Input: dimensioned drawing with shaded views. Units: mm. Origin: part minimum x, y, z. Round coordinates to 2 decimals unless told otherwise and drop trailing zeros. Order: outer loops, then holes, each group sorted by start corner. A loop starts at its lowest first (then second) coordinate and runs counter-clockwise, first axis right, second up.
Item 1: Line query: L1, parallel to Y at x = 81, z = 9.75; L2, parallel to X at y = 5.25, z = 7; L3, parallel to Z at x = 9.5, y = 7. Output: solid intervals per line, ascending.
Item 2: Cut plane C-C on x = 91. Output: boundary loops of the cut face in (y, z).
Item 3: Cut plane A-A on x = 5. Output: boundary loops of the cut face in (y, z).
Item 4: Cut plane B-B on z = 6.5. Output: boundary loops of the cut face in (x, y).
Item 5: First-contact query: pin 1 (2.5 mm diameter, centred on x = 91, y = 5, fed in from -Z); pin 2 (3 mm diameter, centred on x = 26.5, y = 7.5, fed in from +Z). Flat tips, straight axial feed; report the tip coordinate or a pass-through.
Item 6: Mould query, pull axis X, two halves, no side actions, for the marked faces 1, 2 and 3. Classes: released by +X, released by -X, zero draft, split by the parting line, or undercut.
Item 7: Cut plane D-D on y = 2.5. Output: boundary loops of the cut face in (x, z).
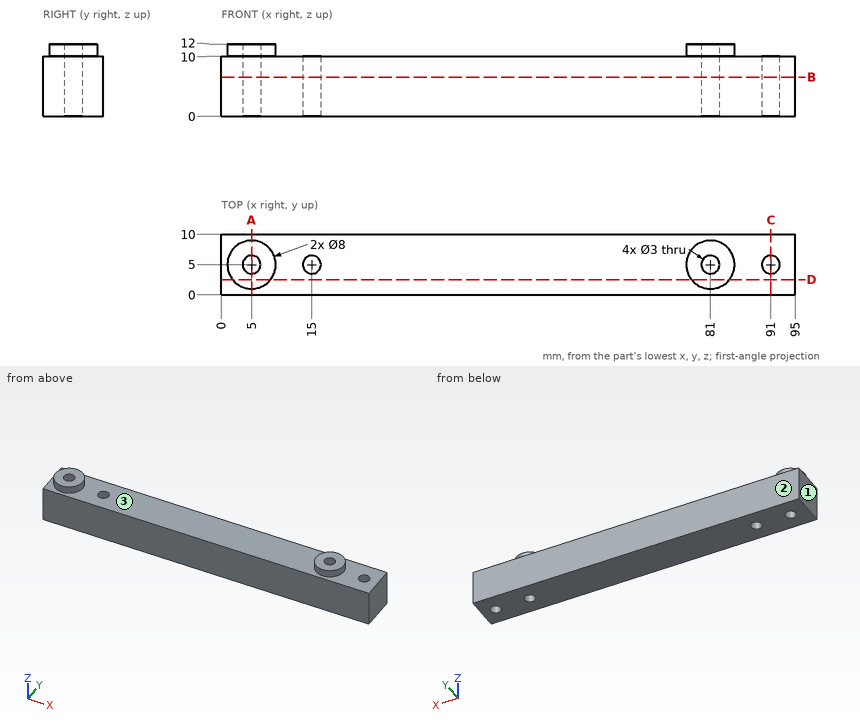
From the geometry:
1. L1: y = 0 to 3.5, 6.5 to 10
1. L2: x = 0 to 3.52, 6.48 to 13.52, 16.48 to 79.52, 82.48 to 89.52, 92.48 to 95
1. L3: z = 0 to 10
2. outline: (0, 0) - (3.5, 0) - (3.5, 10) - (0, 10) - close; (6.5, 0) - (10, 0) - (10, 10) - (6.5, 10) - close
3. outline: (0, 0) - (3.5, 0) - (3.5, 12) - (1, 12) - (1, 10) - (0, 10) - close; (6.5, 0) - (10, 0) - (10, 10) - (9, 10) - (9, 12) - (6.5, 12) - close
4. outline: (0, 0) - (95, 0) - (95, 10) - (0, 10) - close; hole circle Ø3 at (5, 5); hole circle Ø3 at (15, 5); hole circle Ø3 at (81, 5); hole circle Ø3 at (91, 5)
5. pin 1: passes through
5. pin 2: stops at z = 10
6. face 1: released by -X
6. face 2: zero draft
6. face 3: undercut
7. outline: (0, 0) - (95, 0) - (95, 10) - (84.12, 10) - (84.12, 12) - (77.88, 12) - (77.88, 10) - (8.12, 10) - (8.12, 12) - (1.88, 12) - (1.88, 10) - (0, 10) - close
